For this review, take the finished solid that the model builds, in its own axes (mm). Round coordinates to 2 decimals unless told otherwise and drop trailing zeros. Loops run counter-clockwise (first coordinate to the right, second up) from the corner with the lowest first, then second, coordinate; pieces in that order, holes last.
1. Consider section A-A on z = -2.5. State the section outline as (x, y) points, then the cut area to 3 significant figures.
2. Consider section B-B on y = 11. State the section outline as (x, z) points, then the cut area to 3 significant figures.
3. Clearance check with flat-ended pins moving along their axes: pin 1 Ø3 at (x, y) = (-6.5, -9) entering from -Z; pin 2 Ø4 at (x, y) = (0.5, -0.5) entering from +Z; pin 3 Ø10 at (x, y) = (-10, -4.5) entering from +Z. State where each tip first meets the part, or that it passes through.
4. Consider section C-C on y = -7.75. State the section outline as (x, z) points.
5. To check wall thickness, follow line 1 along Z through (x, y) = (-5.5, 12.5); line 2 along Y through (x, z) = (0.5, -10.75); line 3 along Z through (x, y) = (-0.75, 1.75). State the ranges of each line that lie inside material, in increasing order.
6. Consider section D-D on z = 13. State the section outline as (x, y) points.
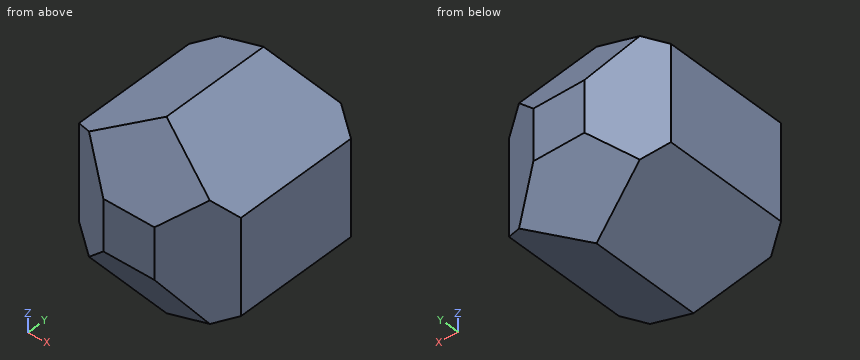
from build123d import *

# Parameters (mm, degrees)
F1_DEPTH = 15
F3_DEPTH = 15
F5_DEPTH = 15


with BuildPart() as f1:
    # F0 (on Top) → F1 (new body, symmetric)
    with BuildSketch(Plane.XY):
        Polygon((14.639726, -9.256264), (15.336023, 8.050243), (0.696296, 17.306507), (-14.639726, 9.256264), (-15.336023, -8.050243), (-0.696296, -17.306507), align=None)
    extrude(amount=F1_DEPTH, both=True)

    # F2 (on Right) → F3 (intersect, symmetric)
    with BuildSketch(Plane.YZ):
        Polygon((8.660254, 15), (-8.660254, 15), (-17.320508, 0), (-8.660254, -15), (8.660254, -15), (17.320508, 0), align=None)
    extrude(amount=F3_DEPTH, both=True, mode=Mode.INTERSECT)

    # F4 (on Front) → F5 (intersect, symmetric)
    with BuildSketch(Plane.XZ):
        Polygon((-12.990381, 7.5), (-12.990381, -7.5), (0, -15), (12.990381, -7.5), (12.990381, 7.5), (0, 15), align=None)
    extrude(amount=F5_DEPTH, both=True, mode=Mode.INTERSECT)


solid = f1.part
Resolved:
1. outline: (-12.99, -9.53) - (-4.34, -15) - (3.7, -15) - (12.99, -10.12) - (12.99, 9.53) - (4.34, 15) - (-3.7, 15) - (-12.99, 10.12) - close
1. area: 687 mm2
2. outline: (-11.32, -8.47) - (-7.02, -10.95) - (7.02, -10.95) - (10.67, -8.84) - (10.67, 8.84) - (7.02, 10.95) - (-7.02, 10.95) - (-11.32, 8.47) - close
2. area: 463 mm2
3. pin 1: stops at z = -12.11
3. pin 2: stops at z = 15
3. pin 3: stops at z = 12.11
4. outline: (-12.99, -7.5) - (0, -15) - (12.99, -7.5) - (12.99, 7.5) - (0, 15) - (-12.99, 7.5) - close
5. line 1: z = -8.35 to 8.35
5. line 2: y = -11.11 to 11.11
5. line 3: z = -14.57 to 14.57
6. outline: (-3.46, -9.81) - (3.46, -9.81) - (3.46, 9.81) - (-3.46, 9.81) - close
